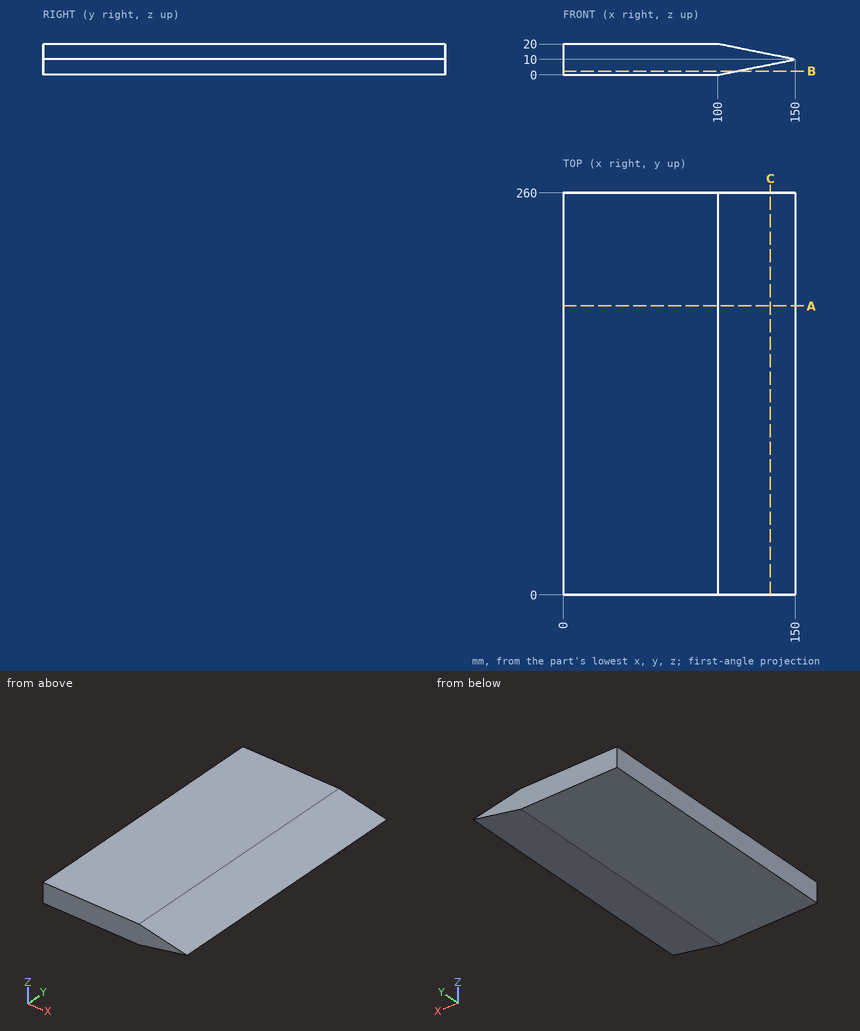
Verification items for this drawing (mm, ordinates from the low corner). Coordinates: 2 decimals unless noted, no trailing zeros. Loops run counter-clockwise (first coordinate to the right, second up) from the corner with the lowest first, then second, coordinate; pieces in that order, holes last. Notation, with made-up numbers: (75, -29) - (133, -29) arc R30 ccw to (133, -7) - close; hole circle Ø1 at (-17, 70). An arc over 180 degrees is marked (long way). One line per item, written item: value. Start each with the question number.
(1) Cross-section at B-B on z = 2.5. Enter the section's corners in (x, y).
(2) Cross-section at C-C on x = 134. Enter the section's corners in (y, z).
(3) Depth check by flat-ended pin: P1, Ø5, axis at x = 124, y = 224, coming from the -Z side. Enter the tip coordinate at first touch or a pass-through.
(4) Cross-section at A-A on y = 187. Enter the section's corners in (x, z).
(5) Material ranges on line 1 (Z direction, x = 122, y = 224); line 2 (Z direction, x = 135, y = 34.5), recorded low to high. Write a range as [from, to].
Results below:
1. outline: (0, 0) - (112.5, 0) - (112.5, 260) - (0, 260) - close
2. outline: (0, 6.8) - (260, 6.8) - (260, 13.2) - (0, 13.2) - close
3. P1: stops at z = 4.3
4. outline: (0, 0) - (100, 0) - (150, 10) - (100, 20) - (0, 20) - close
5. line 1: z = [4.4, 15.6]
5. line 2: z = [7, 13]
